Here's how the part is built. I have some questions about the finished solid (model axes, mm). Face numbers are marked on the shaded views. A direction names the side the tool comes from. Coordinates: 2 decimals unless noted, no trailing zeros. Order: outer loops, then holes, each group sorted by start corner. A loop starts at its lowest first (then second) coordinate and runs counter-clockwise, first axis right, second up. Notation, with made-up numbers: (3, 70) - (39, 70) arc R10 ccw to (39, 82) - close; hole circle Ø7 at (-23.75, 31). An arc over 180 degrees is marked (long way). Answer as CSV lines item,"result". Start each with the question number.
Q1. Thinking about a two-plate mould opening in X: for the marked faces 1, 2 and 3, which applies, released by +X, released by -X, zero draft, split by the parting line, or undercut?
Q2. Suppose I cut it at B-B (z = 3.5). Please give me the cut outline in (x, y) (3 decimals), then the cut area to 3 significant figures.
Q3. I need wall thicknesses on line 1 (Y direction, x = 0, z = 5.5) (3 decimals); line 2 (Z direction, x = -4.5, y = -3.75); line 3 (Y direction, x = -0.75, z = 5.25). Which ranges of each line are inside material? Lowest first, please.
Q4. Suppose I cut it at A-A (x = 0). Please give me the cut outline in (y, z) (3 decimals).
Q5. For pin 1 Ø4 at (x, z) = (7.5, 2.5) entering from -Y; pin 2 Ø1 at (y, z) = (-0.5, 2) entering from -X; pin 3 Ø2 at (x, z) = (6.5, 1) entering from +Y, each with a flat end and sliding along its axis, tell me the tip position at first contact or that it passes through.
Q6. Suppose I cut it at C-C (z = 2.25). Please give me the cut outline in (x, y) (3 decimals).
Q7. For the marked faces 4, 5, 6 and 7, which set-ups out of +Z, -Z, +X, -X, +Y, -Y let a thin tool reach every point of the face, with its end or its side?
Autodesk Inventor part; units mm, degrees
ref_plane "YZ Plane" through (0, 0, 0) normal (1, 0, 0) x (0, 1, 0)
ref_plane "XZ Plane" through (0, 0, 0) normal (0, 1, 0) x (-1, 0, 0)
ref_plane "XY Plane" through (0, 0, 0) normal (0, 0, 1) x (1, 0, 0)
sketch "Boceto1" plane through (0, 0, 0) normal (0, 0, 1) x (1, 0, 0)
  point P0 (0, 0)
sketch "Boceto2" plane through (0, 0, 0) normal (0, 0, 1) x (1, 0, 0)
  circle A0 centre (0, 0) radius 10.5
  dimension "d0" = 21
extrude "Extrusión1" add sketch "Boceto2" along normal blind 1
sketch "Boceto3" plane through (0, 0, 1) normal (0, 0, 1) x (1, 0, 0)
  circle A0 centre (0, 0) radius 3.375
  circle A1 centre (0, 0) radius 5
  line L0 (0, 5) -> (3, 5)
  line L1 (0, 8.6714) -> (0, 6.7493)
  line L2 (0, 5) -> (-3, 5)
  line L3 (-4.3301, 2.5) -> (-2.8301, 5.0981)
  line L4 (-4.3301, 2.5) -> (-5.8301, -0.0981)
  line L5 (-4.3301, -2.5) -> (-5.8301, 0.0981)
  line L6 (-4.3301, -2.5) -> (-2.8301, -5.0981)
  line L7 (0, -5) -> (-3, -5)
  line L8 (0, -5) -> (3, -5)
  line L9 (4.3301, -2.5) -> (2.8301, -5.0981)
  line L10 (4.3301, -2.5) -> (5.8301, 0.0981)
  line L11 (4.3301, 2.5) -> (5.8301, -0.0981)
  line L12 (4.3301, 2.5) -> (2.8301, 5.0981)
  point P0 (-2.8868, 5)
  point P1 (-5.7735, 0)
  point P2 (-2.8868, -5)
  point P3 (2.8868, -5)
  point P4 (5.7735, 0)
  point P5 (2.8868, 5)
  dimension "d4" = 10
  dimension "d3" = 6.75
  dimension "d5" = 3
  dimension "d8" = 360
extrude "Extrusión2" add sketch "Boceto3" along normal blind 7
sketch "Boceto4" plane through (0, 0, 1) normal (0, 0, 1) x (1, 0, 0)
  circle A0 centre (0, 0) radius 10.5
extrude "Extrusión3" add sketch "Boceto4" along normal blind 2
chamfer "Chaflán1" distance 2 angle 45 1 edges at (-10.5, 0, 3)
sketch "Boceto5" plane through (0, 0, 8) normal (0, 0, 1) x (1, 0, 0)
  circle A0 centre (0, 0) radius 3.375
extrude "Extrusión4" cut sketch "Boceto5" against normal blind 8
properties part number "Tuerca para tornillo"
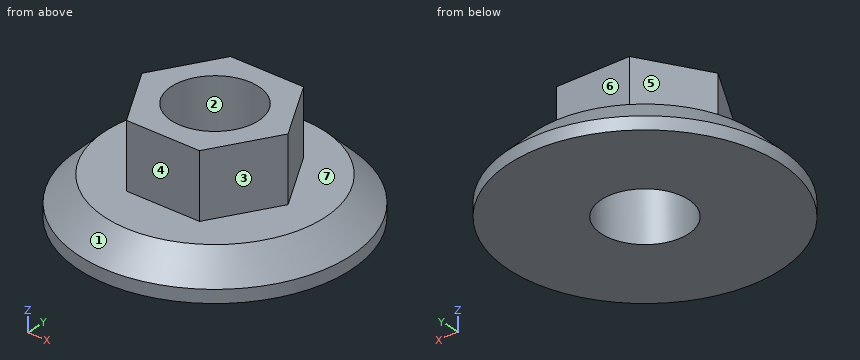
Here are the results:
1,face 1,"split by the parting line"
1,face 2,"undercut"
1,face 3,"released by +X"
2,outline,"(-5.773, 0) - (-2.887, -5) - (2.887, -5) - (5.773, 0) - (2.887, 5) - (-2.887, 5) - close; hole circle Ø6.75 at (0, 0)"
2,area,"50.8 mm²"
3,line 1,"y = -5 to -3.375, 3.375 to 5"
3,line 2,"z = 0 to 3"
3,line 3,"y = -5 to -3.29, 3.29 to 5"
4,outline,"(-10.5, 0) - (-3.375, 0) - (-3.375, 8) - (-5, 8) - (-5, 3) - (-8.5, 3) - (-10.5, 1) - close; (3.375, 0) - (10.5, 0) - (10.5, 1) - (8.5, 3) - (5, 3) - (5, 8) - (3.375, 8) - close"
5,pin 1,"stops at y = -8.49"
5,pin 2,"stops at x = -9.99"
5,pin 3,"stops at y = 8.94"
6,outline,"circle Ø18.5 at (0, 0); hole circle Ø6.75 at (0, 0)"
7,face 4,"+Z, +X, -X, -Y"
7,face 5,"+Z, -X, +Y"
7,face 6,"+Z, +X, -X, +Y"
7,face 7,"+Z"
